Can you work these out from the drawing? Everything is in mm from the part's minimum corner. A direction names the side the tool comes from. Give positions to 0.01 mm unless a question says otherwise; leave off trailing zeros. Loops run counter-clockwise (first coordinate to the right, second up) from the corner with the lowest first, then second, coordinate; pieces in that order, holes last.
Q1. If we section it at B-B (z = 8.3): Please give me the cut outline in (x, y) (3 decimals).
Q2. If we section it at A-A (x = 8.3): Please give me the cut outline in (y, z) (3 decimals), plus the area to 3 significant figures.
Q3. For the marked faces 1, 2, 3, 4 and 5, which set-ups out of +Z, -Z, +X, -X, +Y, -Y let a thin tool reach every point of the face, with its end or its side?
Q4. I need wall thicknesses on line 1 (Z direction, x = 8.25, y = 5); line 2 (X direction, y = 4, z = 7); line 3 (Y direction, x = 3, z = 3.25) (3 decimals). Which ranges of each line are inside material? Lowest first, please.
Q5. If we section it at C-C (y = 17): Please give me the cut outline in (x, z) (3 decimals), plus the area to 3 significant figures.
Q6. If we section it at D-D (z = 14.25): Please give me the cut outline in (x, y) (3 decimals), plus the area to 3 significant figures.
Q7. Will these pins go through, and if not, where does the flat tip stop? P1, Ø5, axis at y = 11.5, z = 8, coming from the -X side; P2, Ø3, axis at y = 32.5, z = 15, coming from the -X side; P3, Ø4, axis at x = 5, y = 18.5, coming from the +Z side.
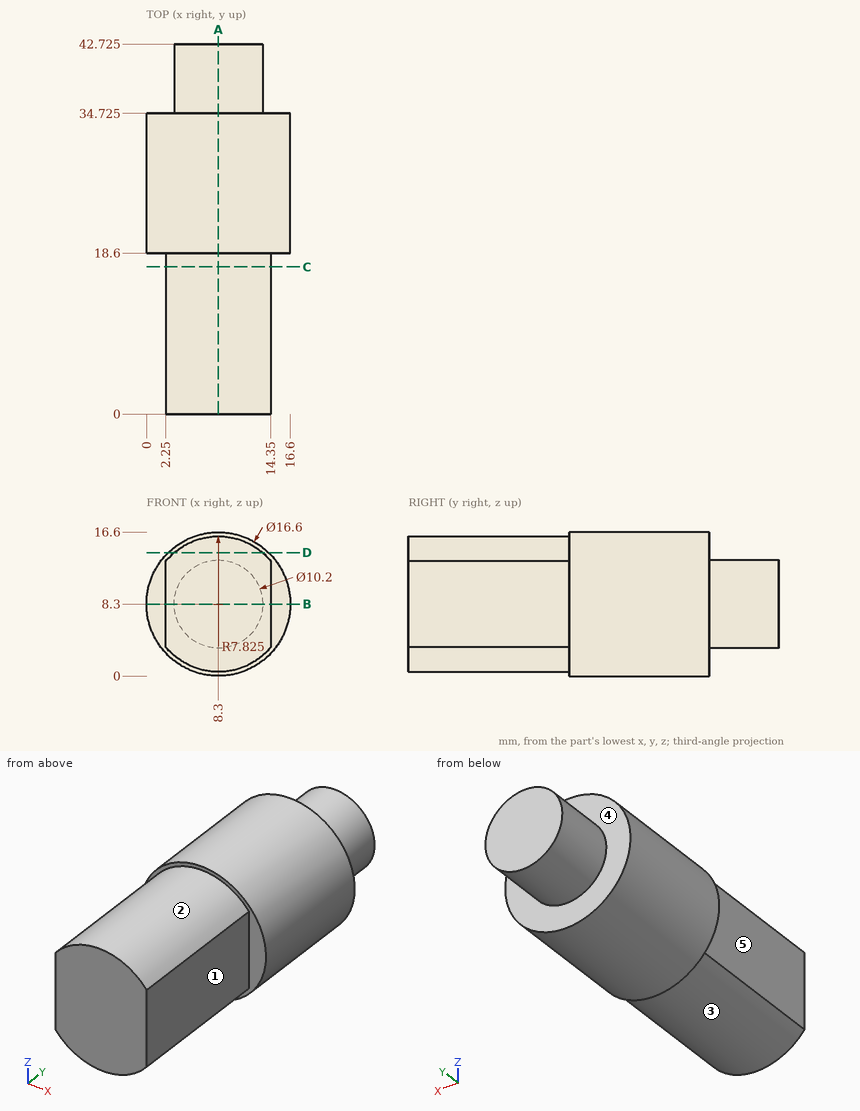
Check sheet entries:
1. outline: (0, 18.6) - (2.25, 18.6) - (2.25, 0) - (14.35, 0) - (14.35, 18.6) - (16.6, 18.6) - (16.6, 34.725) - (13.4, 34.725) - (13.4, 42.725) - (3.2, 42.725) - (3.2, 34.725) - (0, 34.725) - close
2. outline: (0, 0.475) - (18.6, 0.475) - (18.6, 0) - (34.725, 0) - (34.725, 3.2) - (42.725, 3.2) - (42.725, 13.4) - (34.725, 13.4) - (34.725, 16.6) - (18.6, 16.6) - (18.6, 16.125) - (0, 16.125) - close
2. area: 640 mm2
3. face 1: +Z, -Z, +X, -Y
3. face 2: +Z, -Y
3. face 3: -Z, -Y
3. face 4: +Y
3. face 5: +Z, -Z, -X, -Y
4. line 1: z = 0.48 to 16.12
4. line 2: x = 2.25 to 14.35
4. line 3: y = 0 to 34.725
5. outline: (2.25, 3.337) arc R7.825 ccw to (14.35, 3.337) - (14.35, 13.263) arc R7.825 ccw to (2.25, 13.263) - close
5. area: 168 mm2
6. outline: (2.513, 18.6) - (3.218, 18.6) - (3.218, 0) - (13.382, 0) - (13.382, 18.6) - (14.087, 18.6) - (14.087, 34.725) - (2.513, 34.725) - close
6. area: 376 mm2
7. P1: stops at x = 2.25
7. P2: stops at x = 1.83
7. P3: stops at z = 16.5
